```python
from build123d import *

# Parameters (mm, degrees)
F0_R     = 9.525
F1_DEPTH = 76.2
F2_R     = 3.175
F3_DEPTH = 88.9
F4_R     = 2.54


with BuildPart() as f1:
    # F0 (on Front) → F1 (new body)
    with BuildSketch(Plane.XZ):
        Circle(F0_R)
    extrude(amount=-F1_DEPTH)

    # F2 (on Right) → F3 (join)
    with BuildSketch(Plane.YZ):
        with Locations((38.1, 0)):
            Circle(F2_R)
    extrude(amount=F3_DEPTH)

    # F4
    f4_edges = [f1.edges().sort_by_distance(p)[0] for p in [
        (88.9, 34.925, 0),
    ]]
    fillet(f4_edges, radius=F4_R)


solid = f1.part
```
For this review, take the finished solid that the model builds, in its own axes (mm). A direction names the side the tool comes from. Round coordinates to 2 decimals unless told otherwise and drop trailing zeros. Write each loop counter-clockwise with the first axis right and the second up, starting at its lowest first coordinate (ties: lowest second). Pieces come first, ordered by that corner, then holes. Notation, with made-up numbers: (-18.5, 46.25) - (33.5, 46.25) arc R17 cw to (33.5, 78.25) - close; hole circle Ø8 at (73.5, -14.75). An arc over 180 degrees is marked (long way). Answer as a JSON object with one key per item and string values.
1. We need section B-B on y = 20. Give the boundary of the cut face in (x, z) (3 decimals), then the cut area to 3 significant figures.
Response values:
{"outline": "circle Ø19.05 at (0, 0)", "area": "285 mm2"}
2. We need section A-A on x = 59. Give the boundary of the cut face in (y, z) (3 decimals).
Response values:
{"outline": "circle Ø6.35 at (38.1, 0)"}
3. Tool access review of faces 1 (the face through (0, 0, 0)), 2 (the face through (47.13, 34.93, 0.14)): name each direction out of +Z, -Z, +X, -X, +Y, -Y from which nothing blocks a thin tool from reaching the whole face with its end or side.
Response values:
{"face 1": "+Z, -Z, +X, -X, -Y", "face 2": "+X"}
4. We need section D-D on z = -5.75. Give the boundary of the cut face in (x, y), then the cut area to 3 significant figures.
Response values:
{"outline": "(-7.59, 0) - (7.59, 0) - (7.59, 76.2) - (-7.59, 76.2) - close", "area": "1,160 mm2"}
5. For pin 1 Ø1.5 at (x, z) = (71.5, 3.5) entering from +Y; pin 2 Ø2 at (x, y) = (8.5, 61) entering from -Z; pin 3 Ø10 at (x, y) = (6, 47.5) entering from +Z, all flat-tipped, find the tip position at first contact; note any pin that passes through.
Response values:
{"pin 1": "stops at y = 39.69", "pin 2": "stops at z = -5.87", "pin 3": "stops at z = 9.47"}
6. We need section C-C on z = 8. Give the boundary of the cut face in (x, y).
Response values:
{"outline": "(-5.17, 0) - (5.17, 0) - (5.17, 76.2) - (-5.17, 76.2) - close"}
7. To check wall thickness, follow line 1 along X through (y, z) = (7, 0.5); line 2 along Z through (x, y) = (58.5, 39.5); line 3 along X through (y, z) = (16, 6.5). State the ranges of each line that lie inside material, in increasing order.
Response values:
{"line 1": "x = -9.51 to 9.51", "line 2": "z = -2.85 to 2.85", "line 3": "x = -6.96 to 6.96"}
